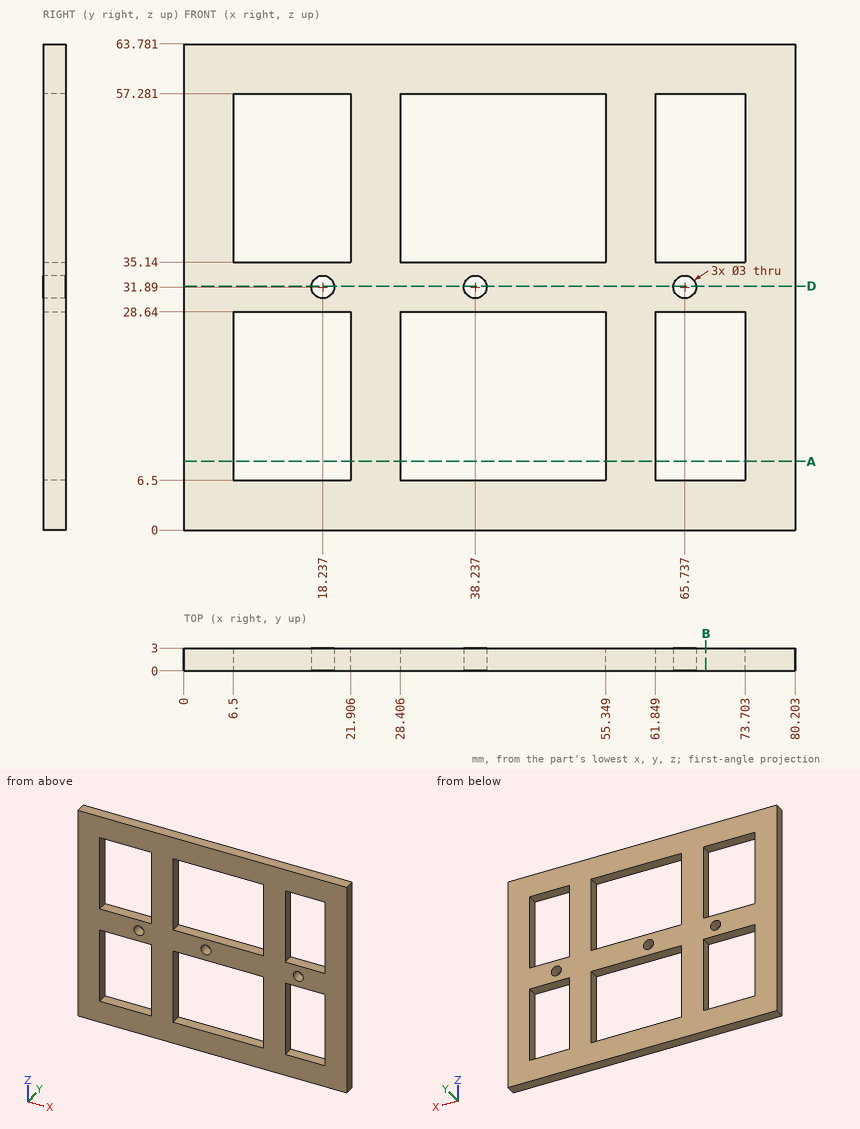
Part print with two shaded views. Sizes in mm from the minimum x, y, z corner. Coordinates: 2 decimals unless noted, no trailing zeros. Loops run counter-clockwise (first coordinate to the right, second up) from the corner with the lowest first, then second, coordinate; pieces in that order, holes last. Notation, with made-up numbers: (87.5, -26) - (93.5, -26) arc R8 ccw to (93.5, -17) - close; hole circle Ø3 at (28.5, 15). An arc over 180 degrees is marked (long way). Write each question's results on one line, items separated by ' | '. Start each with the question number.
Q1. Slice it at A-A on z = 9. Give the number of separate pieces and of enclosed holes in the cut face.
Q2. Slice it at B-B on x = 68.5. Give the cut face in (y, z).
Q3. Probe line 1 along Z through (x, y) = (14.5, 1.3); line 2 along X through (y, z) = (1.5, 33) (1 decimal). List the from-to ranges inside material, lowest first.
Q4. Slice it at D-D on z = 32. Give the cut face in (x, y).
Q5. Drop a flat-ended pin along its axis: pin 1 Ø2.5 at (x, z) = (65.74, 31.89) entering from +Y. Give the stop position or say it passes through.
Answer:
1) separate pieces: 4 | enclosed holes: 0
2) outline: (0, 0) - (3, 0) - (3, 6.5) - (0, 6.5) - close; (0, 28.64) - (3, 28.64) - (3, 35.14) - (0, 35.14) - close; (0, 57.28) - (3, 57.28) - (3, 63.78) - (0, 63.78) - close
3) line 1: z = 0 to 6.5, 28.64 to 35.14, 57.28 to 63.78 | line 2: x = 0 to 17.2, 19.2 to 37.2, 39.2 to 64.7, 66.7 to 80.2
4) outline: (0, 0) - (16.74, 0) - (16.74, 3) - (0, 3) - close; (19.73, 0) - (36.74, 0) - (36.74, 3) - (19.73, 3) - close; (39.73, 0) - (64.24, 0) - (64.24, 3) - (39.73, 3) - close; (67.23, 0) - (80.2, 0) - (80.2, 3) - (67.23, 3) - close
5) pin 1: passes through
